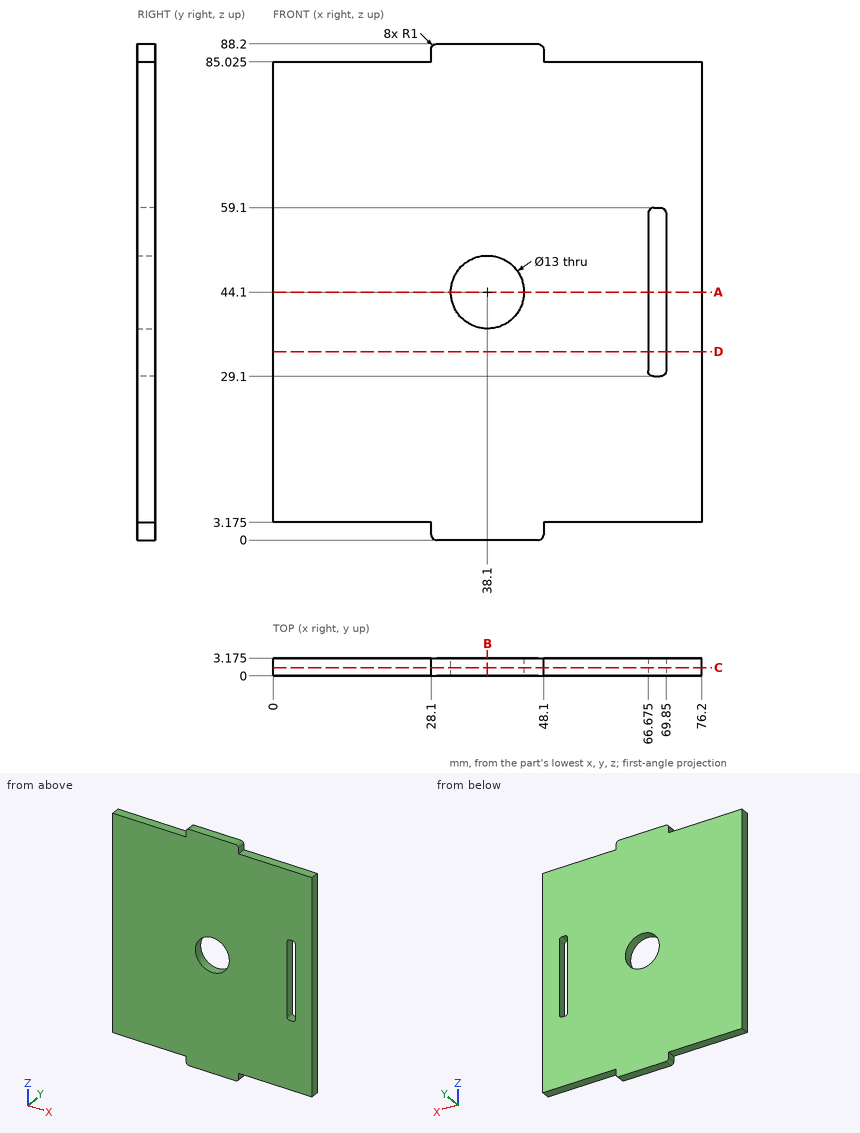
Answer from the drawing. Dimensions are ordinates in mm from the lowest x, y and z of the part. Coordinates: 2 decimals unless noted, no trailing zeros. Write each loop counter-clockwise with the first axis right and the second up, starting at its lowest first coordinate (ties: lowest second). Pieces come first, ordered by that corner, then holes. Notation, with made-up numbers: (29, -8.5) - (34, -8.5) arc R17 cw to (34, 1.5) - close; hole circle Ø10 at (87.5, 32.5). An arc over 180 degrees is marked (long way). Return JSON: item names as keys, results as strings. Group by question number.
Q1. The part is cut by section B-B on x = 38.1. Write down the section's boundary in (y, z) (3 decimals).
Q2. Find the intervals of material crossed by line 1 along Z through (x, y) = (38.1, 1.25); line 2 along X through (y, z) = (1, 44.1) (3 decimals); line 3 along Z through (x, y) = (69, 1.95) (3 decimals), in increasing order. Write a range as [from, to].
Q3. The part is cut by section C-C on y = 1.5. Write down the section's boundary in (x, z) (3 decimals).
Q4. The part is cut by section A-A on z = 44.1. Write down the section's boundary in (x, y) (3 decimals), and give its area (3 significant figures).
Q5. The part is cut by section D-D on z = 33.5. Write down the section's boundary in (x, y) (3 decimals).
Q6. Flat-ended cylindrical pins translate along their axes: pin 1 Ø17 at (x, z) = (38.1, 44.1) entering from -Y; pin 2 Ø1.1 at (y, z) = (1.5, 1.5) entering from +X; pin 3 Ø1.7 at (y, z) = (1, 86.5) entering from -X; pin 4 Ø1.3 at (x, y) = (68.5, 2) entering from -Z (3 decimals). Find the tip coordinate at first contact, or state that the pin passes through.
Evaluation:
{
 "1": {"outline": "(0, 0) - (3.175, 0) - (3.175, 37.6) - (0, 37.6) - close; (0, 50.6) - (3.175, 50.6) - (3.175, 88.2) - (0, 88.2) - close"},
 "2": {"line 1": "z = [0, 37.6], [50.6, 88.2]", "line 2": "x = [0, 31.6], [44.6, 66.675], [69.85, 76.2]", "line 3": "z = [3.175, 29.111], [59.089, 85.025]"},
 "3": {"outline": "(0, 3.175) - (28.1, 3.175) - (28.1, 1) arc R1 ccw to (29.1, 0) - (47.1, 0) arc R1 ccw to (48.1, 1) - (48.1, 3.175) - (76.2, 3.175) - (76.2, 85.025) - (48.1, 85.025) - (48.1, 87.2) arc R1 ccw to (47.1, 88.2) - (29.1, 88.2) arc R1 ccw to (28.1, 87.2) - (28.1, 85.025) - (0, 85.025) - close; hole circle Ø13 at (38.1, 44.1); hole (66.675, 30.1) arc R1 ccw to (67.675, 29.1) - (68.85, 29.1) arc R1 ccw to (69.85, 30.1) - (69.85, 58.1) arc R1 ccw to (68.85, 59.1) - (67.675, 59.1) arc R1 ccw to (66.675, 58.1) - close"},
 "4": {"outline": "(0, 0) - (31.6, 0) - (31.6, 3.175) - (0, 3.175) - close; (44.6, 0) - (66.675, 0) - (66.675, 3.175) - (44.6, 3.175) - close; (69.85, 0) - (76.2, 0) - (76.2, 3.175) - (69.85, 3.175) - close", "area": "191 mm2"},
 "5": {"outline": "(0, 0) - (66.675, 0) - (66.675, 3.175) - (0, 3.175) - close; (69.85, 0) - (76.2, 0) - (76.2, 3.175) - (69.85, 3.175) - close"},
 "6": {"pin 1": "stops at y = 0", "pin 2": "stops at x = 48.1", "pin 3": "stops at x = 28.1", "pin 4": "stops at z = 3.175"}
}
